Autodesk Inventor part; units mm, degrees
ref_plane "YZ Plane" through (0, 0, 0) normal (1, 0, 0) x (0, 1, 0)
ref_plane "XZ Plane" through (0, 0, 0) normal (0, 1, 0) x (-1, 0, 0)
ref_plane "XY Plane" through (0, 0, 0) normal (0, 0, 1) x (1, 0, 0)
sketch "Sketch1" plane through (0, 0, 0) normal (0, 0, 1) x (1, 0, 0)
  line L0 (-50.8, -28.575) -> (50.8, -28.575)
  line L1 (50.8, -28.575) -> (50.8, 28.575)
  line L2 (50.8, 28.575) -> (-50.8, 28.575)
  line L3 (-50.8, 28.575) -> (-50.8, -28.575)
  line L4 (-50.8, -28.575) -> (50.8, 28.575) construction
  line L5 (50.8, -28.575) -> (-50.8, 28.575) construction
  point P0 (0, 0)
  dimension "d0" = 101.6
  dimension "d1" = 57.15
extrude "WR-LEN" add sketch "Sketch1" against normal blind 127
sketch "Sketch2" plane through (0, 0, 0) normal (0, 0, 1) x (1, 0, 0)
  line L0 (3.5309, 20.7371) -> (17.8184, 20.7371)
  line L1 (17.8184, 20.7371) -> (17.8184, 11.2121)
  line L2 (17.8184, 11.2121) -> (3.5309, 11.2121)
  line L3 (3.5309, 11.2121) -> (3.5309, 20.7371)
  line L4 (3.5309, 20.7371) -> (17.8184, 11.2121) construction
  line L5 (17.8184, 20.7371) -> (3.5309, 11.2121) construction
  line L6 (26.1201, 20.7371) -> (40.4265, 20.7371)
  line L7 (40.4265, 20.7371) -> (40.4265, 11.2121)
  line L8 (40.4265, 11.2121) -> (26.1201, 11.2121)
  line L9 (26.1201, 11.2121) -> (26.1201, 20.7371)
  point P0 (0, 0)
  point P1 (10.6746, 15.9746)
  dimension "d4" = 9.525
  dimension "d5" = 14.2875
extrude "sfp ports" cut sketch "Sketch2" against normal blind 12.7
sketch "Sketch3" plane through (0, 0, 0) normal (0, 0, 1) x (1, 0, 0)
  circle A0 centre (-38.1, 0) radius 4.8133
  line L0 (-50.8, 28.575) -> (-50.8, -28.575)
  line L1 (50.8, 28.575) -> (-50.8, 28.575)
  circle A1 centre (-24.13, 0) radius 4.8133
  circle A2 centre (-10.16, 0) radius 4.8133
  point P0 (0, 0)
  dimension "d9" = 9.6266
  dimension "d10" = 12.7
  dimension "d11" = 28.575
  dimension "d14" = 13.97
extrude "Extrusion3" add sketch "Sketch3" along normal blind 2.54
properties part number "WR_LEN"
Check sheet for the modelled part. Datum: model origin and axes. Units: mm. A direction names the side the tool comes from. Coordinates: 2 decimals unless noted, no trailing zeros. Loops run counter-clockwise (first coordinate to the right, second up) from the corner with the lowest first, then second, coordinate; pieces in that order, holes last.
1) Sectioned sample at B-B (y = 13). Record the boundary of the cut face in (x, z).
2) Sectioned sample at A-A (x = -38.1). Record the boundary of the cut face in (y, z) (3 decimals), and give its area (3 significant figures).
3) Sectioned sample at C-C (x = 16). Record the boundary of the cut face in (y, z) (3 decimals).
4) Material ranges on probe 1 along Z at (x, y) = (-5.5, 12); probe 2 along Z at (x, y) = (31.5, 19.5), recorded low to high.
5) Gauge pin test, flat ends, axial feed: pin 1 (10 mm diameter, centred on x = 12.5, y = -19.5, fed in from +Z); pin 2 (5 mm diameter, centred on x = 36.5, y = 14, fed in from +Z). Record the tip position at first contact, or that the pin passes through.
6) Sectioned sample at D-D (y = -3). Record the boundary of the cut face in (x, z), and give its area (3 significant figures).
7) Release check for a two-part mould opening along X. For faces 1 (the face through (-10, 0, 2.54)), 2 (the face through (50.8, 0, -63)), 3 (the face through (33, 11.212, -6)) record: released by +X, released by -X, zero draft, split by the parting line, or undercut.
8) Access from +Z, -Z, +X, -X, +Y, -Y to the whole of each face (thin tool, end or side, straight path). Record for faces 4 (the face through (-1, -28.575, -63)), 5 (the face through (-33.654, 1.844, 1.252)).
Check sheet entries:
1. outline: (-50.8, -127) - (50.8, -127) - (50.8, 0) - (40.43, 0) - (40.43, -12.7) - (26.12, -12.7) - (26.12, 0) - (17.82, 0) - (17.82, -12.7) - (3.53, -12.7) - (3.53, 0) - (-50.8, 0) - close
2. outline: (-28.575, -127) - (28.575, -127) - (28.575, 0) - (4.813, 0) - (4.813, 2.54) - (-4.813, 2.54) - (-4.813, 0) - (-28.575, 0) - close
2. area: 7,280 mm2
3. outline: (-28.575, -127) - (28.575, -127) - (28.575, 0) - (20.737, 0) - (20.737, -12.7) - (11.212, -12.7) - (11.212, 0) - (-28.575, 0) - close
4. probe 1: z = -127 to 0
4. probe 2: z = -127 to -12.7
5. pin 1: stops at z = 0
5. pin 2: stops at z = -12.7
6. outline: (-50.8, -127) - (50.8, -127) - (50.8, 0) - (-6.4, 0) - (-6.4, 2.54) - (-13.92, 2.54) - (-13.92, 0) - (-20.37, 0) - (-20.37, 2.54) - (-27.89, 2.54) - (-27.89, 0) - (-34.34, 0) - (-34.34, 2.54) - (-41.86, 2.54) - (-41.86, 0) - (-50.8, 0) - close
6. area: 13,000 mm2
7. face 1: zero draft
7. face 2: released by +X
7. face 3: undercut
8. face 4: +Z, -Z, +X, -X, -Y
8. face 5: +Z
